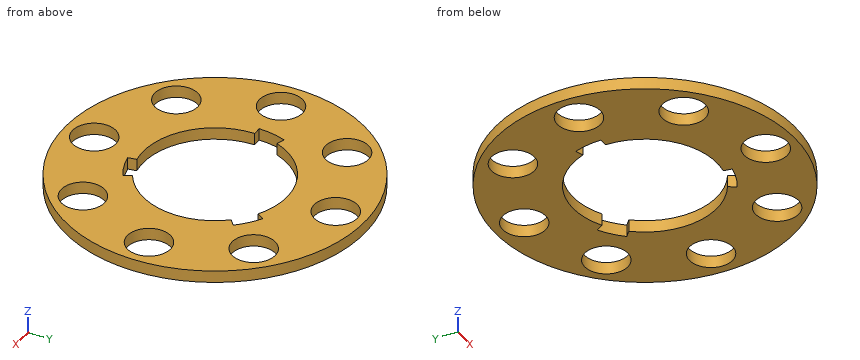
Autodesk Inventor part; units mm, degrees
ref_plane "YZ Plane" through (0, 0, 0) normal (1, 0, 0) x (0, 1, 0)
ref_plane "XZ Plane" through (0, 0, 0) normal (0, 1, 0) x (-1, 0, 0)
ref_plane "XY Plane" through (0, 0, 0) normal (0, 0, 1) x (1, 0, 0)
sketch "Sketch1" plane through (0, 0, 0) normal (0, 0, 1) x (1, 0, 0)
  circle A0 centre (0, 0) radius 100 construction
  circle A1 centre (-100, 0) radius 18
  circle A2 centre (-70.7107, -70.7107) radius 18
  circle A3 centre (0, -100) radius 18
  circle A4 centre (70.7107, -70.7107) radius 18
  circle A5 centre (100, 0) radius 18
  circle A6 centre (70.7107, 70.7107) radius 18
  circle A7 centre (0, 100) radius 18
  circle A8 centre (-70.7107, 70.7107) radius 18
  circle A9 centre (0, 0) radius 125
  circle A10 centre (0, 0) radius 75
  circle A11 centre (0, 0) radius 67.5 construction
  circle A12 centre (0, 0) radius 67
  circle A13 centre (0, 0) radius 60
  line L0 (0, 0) -> (-67, 0)
  line L1 (0, 0) -> (-2.0269, 0)
  line L2 (0, 0) -> (-62.9594, 22.9153)
  line L3 (0, 0) -> (67, 0) construction
  line L4 (0, 0) -> (33.5, -58.0237)
  line L5 (0, 0) -> (11.6344, -65.9821)
  line L6 (0, 0) -> (33.5, 58.0237)
  line L7 (0, 0) -> (51.325, 43.0668)
  point P0 (1.0135, -1.7554)
  point P1 (1.0135, 1.7554)
  point P2 (10.4189, -59.0885)
  point P3 (-60, 0)
  point P4 (-56.3816, 20.5212)
  point P5 (30, 51.9615)
  point P6 (45.9627, 38.5673)
  point P7 (30, -51.9615)
  dimension "d0" = 200
  dimension "d1" = 36
  dimension "d4" = 360
  dimension "d6" = 250
  dimension "d7" = 150
  dimension "d10" = 135
  dimension "d11" = 134
  dimension "d12" = 120
  dimension "d13" = 160
  dimension "d16" = 360
extrude "Extrusion1" add sketch "Sketch1" along normal blind 10 contours A9 | A10 | A12 L4 A13 L7 | L6 A13 L2 A12 | A12 L0 A13 L5
equation "\"d0\" = OuterRadius"
Part model, mm, in its own coordinate system. Coordinates: 2 decimals unless noted, no trailing zeros. Write each loop counter-clockwise with the first axis right and the second up, starting at its lowest first coordinate (ties: lowest second). Pieces come first, ordered by that corner, then holes.
Item 1: Slice it at A-A (x = 100). Write the cut outline in (y, z), and give its area (3 significant figures).
Item 2: Slice it at D-D (z = 4.75). Count the separate pieces of the cut face and the enclosed holes in it, and give its area (3 significant figures).
Item 3: Probe line 1 (Y direction, x = 0, z = 3); line 2 (X direction, y = -69.5, z = 7.75); line 3 (X direction, y = 70, z = 4.75). List the from-to ranges inside material, lowest first.
Item 4: Slice it at C-C (x = 0). Write the cut outline in (y, z), and give its area (3 significant figures).
Item 5: Pin check, flat tips, straight feed: pin 1 (3 mm diameter, centred on y = -53.5, z = 4.5, fed in from +X); pin 2 (6 mm diameter, centred on x = 18.5, z = 3, fed in from +Y); pin 3 (4 mm diameter, centred on x = 56.5, y = -39, fed in from -Z); pin 4 (5 mm diameter, centred on y = 82.5, z = 6, fed in from -X). Stop position of each tip, or through.
Results found:
1. outline: (-75, 0) - (-18, 0) - (-18, 10) - (-75, 10) - close; (18, 0) - (75, 0) - (75, 10) - (18, 10) - close
1. area: 1,140 mm2
2. separate pieces: 1
2. enclosed holes: 9
2. area: 29,200 mm2
3. line 1: y = -125 to -118, -82 to -60, 60 to 82, 118 to 125
3. line 2: x = -103.9 to -88.67, -52.75 to 52.75, 88.67 to 103.9
3. line 3: x = -103.56 to -88.7, -52.72 to 52.72, 88.7 to 103.56
4. outline: (-125, 0) - (-118, 0) - (-118, 10) - (-125, 10) - close; (-82, 0) - (-60, 0) - (-60, 10) - (-82, 10) - close; (60, 0) - (82, 0) - (82, 10) - (60, 10) - close; (118, 0) - (125, 0) - (125, 10) - (118, 10) - close
4. area: 580 mm2
5. pin 1: stops at x = 113.67
5. pin 2: stops at y = 124.04
5. pin 3: stops at z = 0
5. pin 4: stops at x = -96.05
